Here's the drawing with two shaded views (mm, measured from the low corner). I have some questions. A direction names the side the tool comes from. Coordinates: 2 decimals unless noted, no trailing zeros. Write each loop counter-clockwise with the first axis right and the second up, starting at its lowest first coordinate (ties: lowest second). Pieces come first, ordered by that corner, then holes.
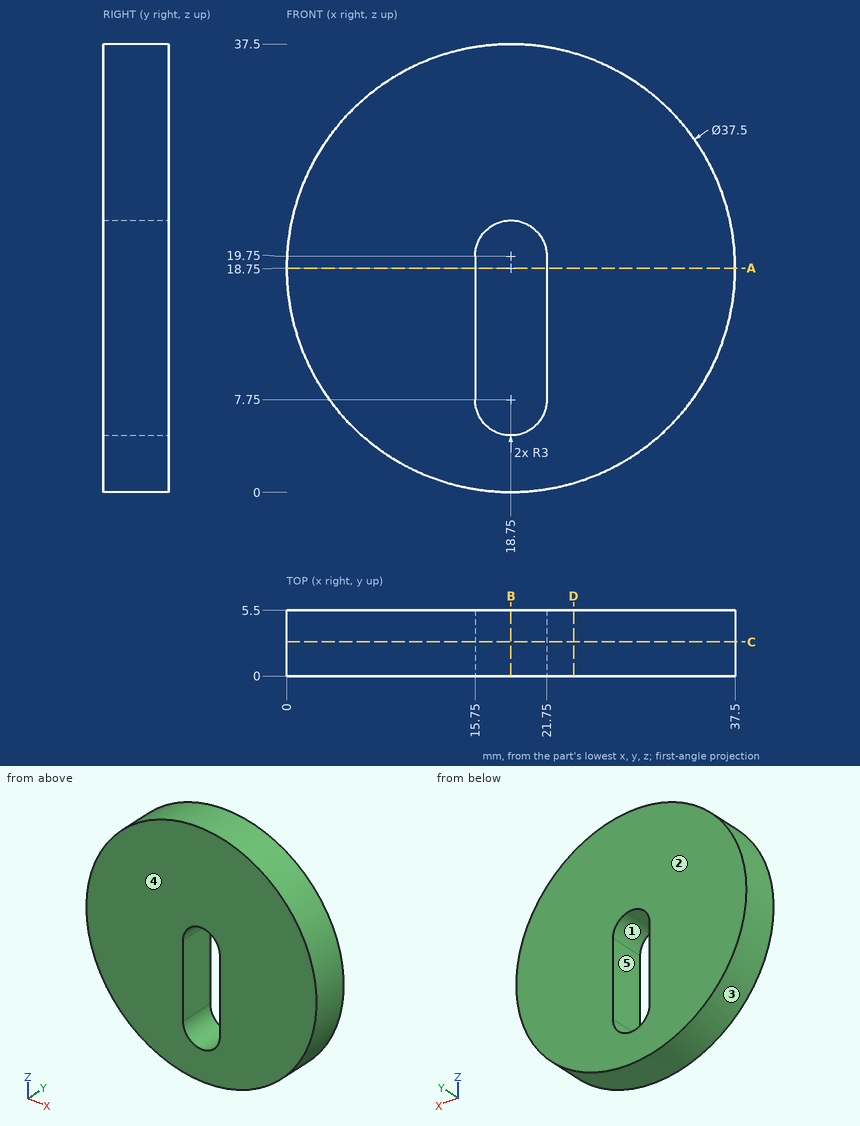
Item 1: Which directions (+Z, -Z, +X, -X, +Y, -Y) give clear straight access to the entire face, cutting with the end or side of a thin tool? Please do the marked faces 4 and 5.
Item 2: I want a section at C-C, the plane y = 2.85. List the corners of the cut face in (x, z) for me.
Item 3: If I drill on line 1 along X through (y, z) = (4, 14); line 2 along Z through (x, y) = (16, 4.35); line 3 along X through (y, z) = (2.4, 18) (3 decimals), over which ranges is the centre line in solid material (lowest first)?
Item 4: I want a section at A-A, the plane z = 18.75. List the corners of the cut face in (x, y) for me.
Item 5: I want a section at B-B, the plane x = 18.75. List the corners of the cut face in (y, z) for me.
Item 6: I want a section at D-D, the plane x = 24. List the corners of the cut face in (y, z) for me.
Item 7: Will these pins go through, and if not, where does the flat tip stop? pin 1 Ø2 at (x, y) = (10, 3.5) entering from +Z; pin 2 Ø3 at (y, z) = (2.5, 14) entering from +X; pin 3 Ø1 at (y, z) = (1.5, 5.5) entering from -X.
Item 8: If we mould it in two halves opening along X, with no side actions, what happens to the marked faces 1, 2 and 3? For each: released by +X, released by -X, zero draft, split by the parting line, or undercut.
Taken from the geometry:
1. face 4: +Z, -Z, +X, -X, -Y
1. face 5: +Y, -Y
2. outline: circle Ø37.5 at (18.75, 18.75); hole (15.75, 7.75) arc R3 ccw to (21.75, 7.75) - (21.75, 19.75) arc R3 ccw to (15.75, 19.75) - close
3. line 1: x = 0.61 to 15.75, 21.75 to 36.89
3. line 2: z = 0.2 to 6.55, 20.95 to 37.3
3. line 3: x = 0.015 to 15.75, 21.75 to 37.485
4. outline: (0, 0) - (15.75, 0) - (15.75, 5.5) - (0, 5.5) - close; (21.75, 0) - (37.5, 0) - (37.5, 5.5) - (21.75, 5.5) - close
5. outline: (0, 0) - (5.5, 0) - (5.5, 4.75) - (0, 4.75) - close; (0, 22.75) - (5.5, 22.75) - (5.5, 37.5) - (0, 37.5) - close
6. outline: (0, 0.75) - (5.5, 0.75) - (5.5, 36.75) - (0, 36.75) - close
7. pin 1: stops at z = 35.82
7. pin 2: stops at x = 37.22
7. pin 3: stops at x = 5
8. face 1: undercut
8. face 2: zero draft
8. face 3: split by the parting line
